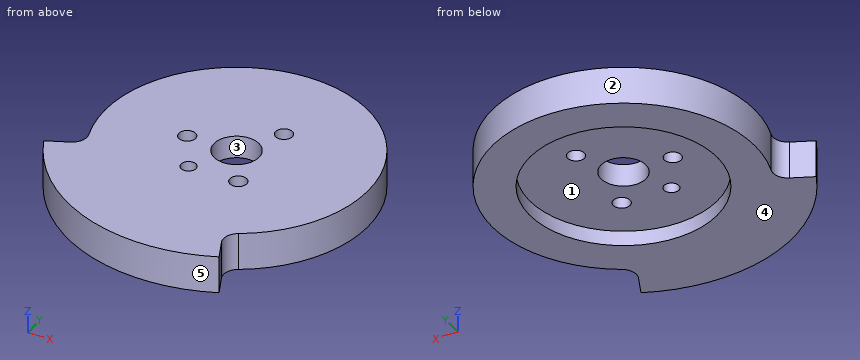
```python
from build123d import *

# Parameters (mm, degrees)
ESQUISSE1_R             = 2.25
ESQUISSE1_R_2           = 6
ESQUISSE1_R_3           = 2
EXTRUSION1_DEPTH        = 10
ESQUISSE2_R             = 25
ENL_V_MAT_EXTRU_1_DEPTH = 4


with BuildPart() as part:
    # Esquisse1 → Extrusion1 (new body)
    with BuildSketch(Plane.XY):
        with BuildLine():
            Line((15.158152138, -35.710368575), (17.582900782, -41.422718405))
            ThreePointArc((17.582900782, -41.422718405), (-16.857296704, -41.723273456), (-41.422718405, -17.582900782))
            Line((-41.422718405, -17.582900782), (-35.710368575, -15.158152138))
            ThreePointArc((-35.710368575, -15.158152138), (-33.646394386, -13.163025073), (-33.450391234, -10.29909347))
            ThreePointArc((-33.450391234, -10.29909347), (13.11123077, 32.45143491), (16.907846264, -30.645142106))
            ThreePointArc((16.907846264, -30.645142106), (15.059385072, -32.841437324), (15.158152138, -35.710368575))
        make_face()
        with Locations((-13, 0)):
            Circle(ESQUISSE1_R, mode=Mode.SUBTRACT)
        with Locations((6.5, 11.258330249)):
            Circle(ESQUISSE1_R, mode=Mode.SUBTRACT)
        with Locations((6.5, -11.258330249)):
            Circle(ESQUISSE1_R, mode=Mode.SUBTRACT)
        Circle(ESQUISSE1_R_2, mode=Mode.SUBTRACT)
        with Locations((-6.670127311, -11.158378093)):
            Circle(ESQUISSE1_R_3, mode=Mode.SUBTRACT)
    extrude(amount=EXTRUSION1_DEPTH)

    # Esquisse2 → Enlèv. mat.-Extru.1 (cut)
    with BuildSketch(Plane(origin=(0, 0, 0), x_dir=(-1, 0, 0), z_dir=(0, 0, -1))):
        Circle(ESQUISSE2_R)
    extrude(amount=-ENL_V_MAT_EXTRU_1_DEPTH, mode=Mode.SUBTRACT)


solid = part.part
```
CAD build for the part. Positions are in the model's coordinates, mm. Face numbers are marked on the shaded views. A direction names the side the tool comes from. Round coordinates to 2 decimals unless told otherwise and drop trailing zeros. Order: outer loops, then holes, each group sorted by start corner. A loop starts at its lowest first (then second) coordinate and runs counter-clockwise, first axis right, second up.
Item 1: Saw through at C-C on z = 7.5. Write the cut outline in (x, y), then the cut area to 3 significant figures.
Item 2: Tool access for the marked faces 1 and 2: list every direction of +Z, -Z, +X, -X, +Y, -Y with a clear straight run to the whole face (end or side of a thin tool).
Item 3: Saw through at D-D on z = 2. Write the cut outline in (x, y), then the cut area to 3 significant figures.
Item 4: Saw through at B-B on x = 0. Write the cut outline in (y, z), then the cut area to 3 significant figures.
Item 5: Saw through at A-A on y = 0. Write the cut outline in (x, z).
Item 6: Pin check, flat tips, straight feed: pin 1 (1.5 mm diameter, centred on x = 12.5, z = 2, fed in from +Y); pin 2 (3 mm diameter, centred on x = -1, y = -13, fed in from -Z); pin 3 (6 mm diameter, centred on y = 26.5, z = 2, fed in from -X); pin 4 (3.5 mm diameter, centred on x = 6.5, y = -11.26, fed in from -Z). Stop position of each tip, or through.
Item 7: Mould opens along Y. For the marked faces 3, 4 and 5 say: pulls with the +Y half, pulls with the -Y half, needs draft (parallel to the pull), parting line crosses it, or undercut.
Item 8: Probe line 1 along X through (y, z) = (0, 8.15); line 2 along Y through (x, z) = (0, 1.1); line 3 along Y through (x, z) = (17, 1.25). List the from-to ranges inside material, lowest first.
Reported:
1. outline: (-41.42, -17.58) arc R45 ccw to (17.58, -41.42) - (15.16, -35.71) arc R4 cw to (16.91, -30.65) arc R35 ccw (long way) to (-33.45, -10.3) arc R4 cw to (-35.71, -15.16) - close; hole circle Ø4.5 at (-13, 0); hole circle Ø4 at (-6.67, -11.16); hole circle Ø12 at (0, 0); hole circle Ø4.5 at (6.5, -11.26); hole circle Ø4.5 at (6.5, 11.26)
1. area: 4,310 mm2
2. face 1: -Z
2. face 2: +Z, -Z
3. outline: (-41.42, -17.58) arc R45 ccw to (17.58, -41.42) - (15.16, -35.71) arc R4 cw to (16.91, -30.65) arc R35 ccw (long way) to (-33.45, -10.3) arc R4 cw to (-35.71, -15.16) - close; hole circle Ø50 at (0, 0)
3. area: 2,520 mm2
4. outline: (-45, 0) - (-25, 0) - (-25, 4) - (-6, 4) - (-6, 10) - (-45, 10) - close; (6, 4) - (25, 4) - (25, 0) - (35, 0) - (35, 10) - (6, 10) - close
4. area: 528 mm2
5. outline: (-35, 0) - (-25, 0) - (-25, 4) - (-15.25, 4) - (-15.25, 10) - (-35, 10) - close; (-10.75, 4) - (-6, 4) - (-6, 10) - (-10.75, 10) - close; (6, 4) - (25, 4) - (25, 0) - (35, 0) - (35, 10) - (6, 10) - close
6. pin 1: stops at y = 32.97
6. pin 2: stops at z = 4
6. pin 3: stops at x = -25.94
6. pin 4: passes through
7. face 3: undercut
7. face 4: needs draft
7. face 5: pulls with the -Y half
8. line 1: x = -35 to -15.25, -10.75 to -6, 6 to 35
8. line 2: y = -45 to -25, 25 to 35
8. line 3: y = -41.67 to -40.05, -30.59 to -18.33, 18.33 to 30.59
